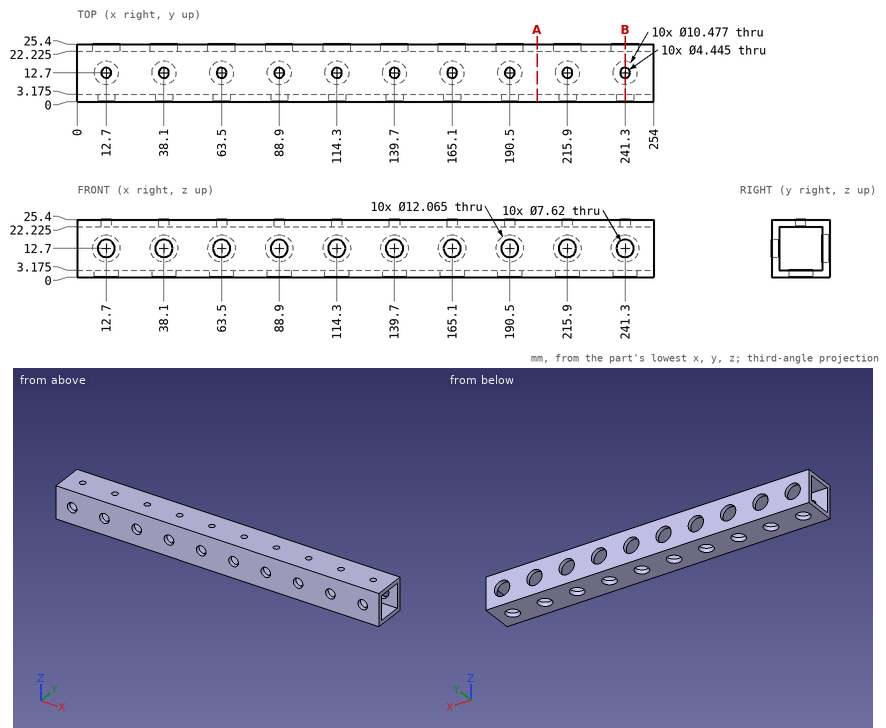
Study the drawing (mm; zero at the part's minimum x, y, z) and answer. Coordinates: 2 decimals unless noted, no trailing zeros. Write each loop counter-clockwise with the first axis right and the second up, starting at its lowest first coordinate (ties: lowest second). Pieces come first, ordered by that corner, then holes. Notation, with made-up numbers: M 19.5,30 L 29.5,30 A23 cw 29.5,47 Z; hole C 66,-9 d7. An arc over 180 degrees is marked long. Use one line per item in the form item = value.
Item 1: Given P1, Ø5, axis at x = 241.3, y = 12.7, coming from the -Z side (1 decimal), flat-ended and moving along its own axis, determine where the tip first touches the part or whether it passes through.
Model answer:
P1 = 22.2
Item 2: Find section A-A, the plane x = 202.5. Give the vertices of the cut face in (y, z) (1 decimal), plus the area to 3 significant figures.
Model answer:
outline = M 0,0 L 25.4,0 L 25.4,25.4 L 0,25.4 Z; hole M 3.2,3.2 L 22.2,3.2 L 22.2,22.2 L 3.2,22.2 Z
area = 282 mm2
Item 3: Find the intervals of material crossed by probe 1 along Z at (x, y) = (90.5, 5.25) (1 decimal); probe 2 along Y at (x, z) = (88.9, 23.25); probe 3 along Z at (x, y) = (241.3, 23.05), in increasing order.
Model answer:
probe_1 = 0 to 3.2, 22.2 to 25.4
probe_2 = 0 to 10.48, 14.92 to 25.4
probe_3 = 0 to 6.67, 18.73 to 25.4
Item 4: Find section B-B, the plane x = 241.3. Give the vertices of the cut face in (y, z) (1 decimal).
Model answer:
outline = M 0,0 L 7.5,0 L 7.5,3.2 L 3.2,3.2 L 3.2,8.9 L 0,8.9 Z; M 0,16.5 L 3.2,16.5 L 3.2,22.2 L 10.5,22.2 L 10.5,25.4 L 0,25.4 Z; M 14.9,22.2 L 22.2,22.2 L 22.2,18.7 L 25.4,18.7 L 25.4,25.4 L 14.9,25.4 Z; M 17.9,0 L 25.4,0 L 25.4,6.7 L 22.2,6.7 L 22.2,3.2 L 17.9,3.2 Z
